Autodesk Inventor part; units mm, degrees
ref_plane "YZ Plane" through (0, 0, 0) normal (1, 0, 0) x (0, 1, 0)
ref_plane "XZ Plane" through (0, 0, 0) normal (0, 1, 0) x (-1, 0, 0)
ref_plane "XY Plane" through (0, 0, 0) normal (0, 0, 1) x (1, 0, 0)
sketch "Sketch1" plane through (0, 0, 0) normal (0, 1, 0) x (-1, 0, 0)
  circle A0 centre (0, 0) radius 25
  circle A1 centre (0, 0) radius 22.5
  circle A2 centre (0, 0) radius 2.25
  line L0 (10, 10) -> (-10, 10)
  line L1 (-10, 10) -> (-10, -10)
  line L2 (-10, -10) -> (10, -10)
  line L3 (10, -10) -> (10, 10)
  line L4 (10, 10) -> (-10, -10) construction
  line L5 (-10, 10) -> (10, -10) construction
  circle A3 centre (10, -10) radius 2.5
  circle A4 centre (-10, -10) radius 2.5
  circle A5 centre (-10, 10) radius 2.5
  circle A6 centre (10, 10) radius 2.5
  circle A7 centre (0, 0) radius 5
  circle A8 centre (0, 0) radius 2.5
  circle A9 centre (0, 0) radius 1
  dimension "d0" = 50
  dimension "d1" = 45
  dimension "d2" = 4.5
  dimension "d3" = 20
  dimension "d4" = 20
  dimension "d5" = 5
  dimension "d6" = 5
  dimension "d7" = 5
  dimension "d8" = 5
  dimension "d27" = 10
  dimension "d28" = 5
  dimension "d29" = 2
extrude "Extrusion1" add sketch "Sketch1" along normal blind 2 contours A2 | A8
sketch "Sketch5" plane through (0, 2, 0) normal (0, 1, 0) x (1, 0, 0)
  circle A0 centre (0, 0) radius 5
  line L0 (-5, 0) -> (-3.2679, 1)
  line L1 (-5, 0) -> (-3, 0) construction
  line L2 (-3.2679, 1) -> (-2.2913, 1)
  circle A1 centre (0, 0) radius 2.5
  line L3 (-5, 0) -> (-3.2679, -1)
  line L4 (-5, 0) -> (-3, 0) construction
  line L5 (-3.2679, -1) -> (-2.2913, -1)
  dimension "d30" = 10
  dimension "d31" = 2
  dimension "d32" = 30
  dimension "d33" = 2
  dimension "d34" = 30
extrude "Extrusion4" add sketch "Sketch5" along normal blind 0.5 and the other way blind 2.5 contours L0 L2 A1 L5 L3
pattern_circular "Circular Pattern2" count 10 over 360 about axis through (0, 0, 0) along (0, 1, 0) of "Extrusion4"
sketch "Sketch6" plane through (0, 2, 0) normal (0, 1, 0) x (1, 0, 0)
  line L0 (1.5451, 4.7553) -> (1.9609, 2.799)
  circle A0 centre (0, 0) radius 5
equation "\"BendRadius\" = Thickness"
equation "\"BendReliefWidth\" = Thickness"
equation "\"BendReliefDepth\" = 0.5 * Thickness"
equation "\"CornerReliefSize\" = 4 * Thickness"
equation "\"MinimumRemnant\" = 2 * Thickness"
equation "\"TransitionRadius\" = BendRadius"
equation "\"JacobiRadiusSize\" = BendRadius"
equation "\"GapSize\" = Thickness"
Part model, mm, in its own coordinate system. A direction names the side the tool comes from. Give positions to 0.01 mm unless a question says otherwise; leave off trailing zeros. Loops run counter-clockwise (first coordinate to the right, second up) from the corner with the lowest first, then second, coordinate; pieces in that order, holes last. Notation, with made-up numbers: M 16,-3 L 74,-3 A29 ccw 74,35 Z; hole C 42,-33.75 d10. An arc over 180 degrees is marked long. Return JSON: item names as keys, results as strings.
1) Flat gauge pins, fed straight in: pin 1 Ø1.5 at (x, z) = (-1, -1) entering from -Y; pin 2 Ø3 at (x, z) = (0, 0) entering from +Y; pin 3 Ø1.2 at (x, z) = (0, 0) entering from -Y. Where does each tip first touch, or does it go through?
Calculated:
{"pin 1": "stops at y = 0", "pin 2": "stops at y = 2", "pin 3": "passes through"}
2) Drill centre lines: line 1 (Z direction, x = -3.75, y = 0); line 2 (X direction, y = 0.1, z = -0.5); line 3 (Y direction, x = 0.75, z = -1.5). Where is each one in solid material? Low to high.
Calculated:
{"line 1": "z = -2.91 to -2.28, -0.72 to 0.72, 2.28 to 2.91", "line 2": "x = -4.13 to -0.87, 0.87 to 4.13", "line 3": "y = 0 to 2"}
3) 3-axis set-ups, long thin cutter, end or side, ignore diameter. For faces 1 (the face through (-1, 0, -1)), 2 (the face through (-3.644, 0.979, -2.038)), 3 (the face through (-3.064, 0.979, -2.836)), 4 (the face through (4.15, 0.98, -0.49)): which of +Z, -Z, +X, -X, +Y, -Y reach the whole face in a straight line?
Calculated:
{"face 1": "-Y", "face 2": "-X, +Y, -Y", "face 3": "-Z, +Y, -Y", "face 4": "+X, +Y, -Y"}
4) Saw through at A-A, the plane z = 4. List the corners of the cut face in (x, y).
Calculated:
{"outline": "M -1.71,-0.5 L -0.71,-0.5 L -0.71,2.5 L -1.71,2.5 Z; M 0.71,-0.5 L 1.71,-0.5 L 1.71,2.5 L 0.71,2.5 Z"}
5) Saw through at D-D, the plane z = -0.75. List the corners of the cut face in (x, y), then the cut area to 3 significant figures.
Calculated:
{"outline": "M -3.7,-0.5 L -2.38,-0.5 L -2.38,0 L -0.66,0 L -0.66,2 L -2.38,2 L -2.38,2.5 L -3.7,2.5 Z; M 0.66,0 L 2.38,0 L 2.38,-0.5 L 3.7,-0.5 L 3.7,2.5 L 2.38,2.5 L 2.38,2 L 0.66,2 Z", "area": "14.8 mm2"}
6) Saw through at B-B, the plane z = 0.25. List the corners of the cut face in (x, y).
Calculated:
{"outline": "M -4.57,-0.5 L -2.49,-0.5 L -2.49,0 L -0.97,0 L -0.97,2 L -2.49,2 L -2.49,2.5 L -4.57,2.5 Z; M 0.97,0 L 2.49,0 L 2.49,-0.5 L 4.57,-0.5 L 4.57,2.5 L 2.49,2.5 L 2.49,2 L 0.97,2 Z"}
7) Pull direction Z, two halves, no side cores. Call faces 5 (the face through (-3.644, 0.979, 2.038)), 6 (the face through (-2, -0.5, 2)), 7 (the face through (-4.15, 0.98, -0.49)), 8 (the face through (0.812, 0.979, 4.095)): released by +Z, released by -Z, zero draft, split by the parting line, or undercut.
Calculated:
{"face 5": "undercut", "face 6": "zero draft", "face 7": "undercut", "face 8": "released by +Z"}
8) Saw through at C-C, the plane x = 2.75. List the corners of the cut face in (y, z), then the cut area to 3 significant figures.
Calculated:
{"outline": "M -0.5,-2.8 L 2.5,-2.8 L 2.5,2.8 L -0.5,2.8 Z", "area": "16.8 mm2"}
